from build123d import *

# Parameters (mm, degrees)
CROQUIS1_W              = 138
CROQUIS1_H              = 53
SALIENTE_EXTRUIR1_DEPTH = 5
CROQUIS2_R              = 2.003620998
CROQUIS2_R_2            = 1.5
CROQUIS2_R_3            = 1.25
PRINCIPAL_DEPTH         = 5
CORTAR_EXTRUIR2_DEPTH   = 5
SALIENTE_EXTRUIR2_DEPTH = 5
CORTAR_EXTRUIR3_DEPTH   = 4
CROQUIS6_R              = 4
CORTAR_EXTRUIR4_DEPTH   = 4
SALIENTE_EXTRUIR3_START = 1
CROQUIS8_R              = 1.25
SALIENTE_EXTRUIR3_DEPTH = 1
CROQUIS9_R              = 1
CORTAR_EXTRUIR5_DEPTH   = 10
CROQUIS10_R             = 1
CORTAR_EXTRUIR6_DEPTH   = 10


with BuildPart() as part:
    # Croquis1 → Saliente-Extruir1 (new body)
    with BuildSketch(Plane.XY):
        Rectangle(CROQUIS1_W, CROQUIS1_H)
    extrude(amount=SALIENTE_EXTRUIR1_DEPTH)

    # Croquis2 → Principal (cut)
    with BuildSketch(Plane.XY.offset(5)):
        Polygon((-27.5, -16.5), (-32.5, 10.5), (-27.5, 24.5), (27.5, 24.5), (32.5, 10.5), (27.5, -16.5), align=None)
        with BuildLine():
            Line((-33.613106132, 13.32973033), (-28.909438392, 26.5))
            Line((-28.909438392, 26.5), (-69, 26.5))
            Line((-69, 26.5), (-69, -26.5))
            Line((-69, -26.5), (-29.659776055, -26.5))
            Line((-29.659776055, -26.5), (-46.481481481, 5))
            Line((-46.481481481, 5), (-59.600761168, 5))
            Line((-59.600761168, 5), (-68.394256163, 20.706415948))
            Line((-68.394256163, 20.706415948), (-65.993243243, 22.505064597))
            Line((-65.993243243, 22.505064597), (-57, 10.5))
            Line((-57, 10.5), (-38.5, 10.5))
            ThreePointArc((-38.5, 10.5), (-37, 12), (-35.5, 10.5))
            Line((-35.5, 10.5), (-35.5, 12))
            ThreePointArc((-35.5, 12), (-36.916773994, 15.420394992), (-33.496379002, 14.003620998))
            ThreePointArc((-33.496379002, 14.003620998), (-33.525776447, 13.661658334), (-33.613106132, 13.32973033))
        make_face()
        with BuildLine():
            Line((28.909438392, 26.5), (33.613106132, 13.32973033))
            ThreePointArc((33.613106132, 13.32973033), (35.158037336, 15.977844551), (37.503620998, 14.003620998))
            ThreePointArc((37.503620998, 14.003620998), (36.916773994, 12.586847003), (35.5, 12))
            Line((35.5, 12), (35.5, 10.5))
            ThreePointArc((35.5, 10.5), (37, 12), (38.5, 10.5))
            Line((38.5, 10.5), (57, 10.5))
            Line((57, 10.5), (65.993243243, 22.505064597))
            Line((65.993243243, 22.505064597), (68.394256163, 20.706415948))
            Line((68.394256163, 20.706415948), (59.600761168, 5))
            Line((59.600761168, 5), (46.481481481, 5))
            Line((46.481481481, 5), (29.659776055, -26.5))
            Line((29.659776055, -26.5), (69, -26.5))
            Line((69, -26.5), (69, 26.5))
            Line((69, 26.5), (28.909438392, 26.5))
        make_face()
        with Locations((-35.5, 14.003620998)):
            Circle(CROQUIS2_R)
        with Locations((35.5, 14.003620998)):
            Circle(CROQUIS2_R)
        with Locations((37, 10.5)):
            Circle(CROQUIS2_R_2)
        with Locations((-37, 10.5)):
            Circle(CROQUIS2_R_2)
        with Locations((-6, -21.25)):
            Circle(CROQUIS2_R_3)
        with Locations((6, -21.25)):
            Circle(CROQUIS2_R_3)
    extrude(amount=-PRINCIPAL_DEPTH, mode=Mode.SUBTRACT)

    # Croquis3 → Cortar-Extruir2 (cut)
    with BuildSketch(Plane.XY.offset(5)):
        with BuildLine():
            ThreePointArc((32.325878128, -21.50750886), (28.853998723, -25.156220871), (24, -26.5))
            Line((24, -26.5), (29.659776055, -26.5))
            Line((29.659776055, -26.5), (32.325878128, -21.50750886))
        make_face()
        with BuildLine():
            ThreePointArc((60.578021878, 6.745524755), (59.326103094, 5.468546056), (57.600287393, 5))
            Line((57.600287393, 5), (59.600761168, 5))
            Line((59.600761168, 5), (60.578021878, 6.745524755))
        make_face()
        with BuildLine():
            Line((28.909438392, 26.5), (27.147640402, 26.5))
            ThreePointArc((27.147640402, 26.5), (28.587761459, 26.043538926), (29.501995152, 24.840841072))
            Line((29.501995152, 24.840841072), (28.909438392, 26.5))
        make_face()
    cortar_extruir2 = extrude(amount=-CORTAR_EXTRUIR2_DEPTH, mode=Mode.SUBTRACT)

    # Simetría2: Cortar-Extruir2 across plane
    add(cortar_extruir2.mirror(Plane(origin=(0, 0, 0), x_dir=(0, 0, 1), z_dir=(1, 0, 0))), mode=Mode.SUBTRACT)

    # Croquis4 → Saliente-Extruir2 (add)
    with BuildSketch(Plane.XY.offset(5)):
        with BuildLine():
            ThreePointArc((27.651464932, -15.682089366), (27.30767909, -16.268794305), (26.668182947, -16.5))
            Line((26.668182947, -16.5), (27.5, -16.5))
            Line((27.5, -16.5), (27.651464932, -15.682089366))
        make_face()
        with BuildLine():
            ThreePointArc((26.795280804, 24.5), (27.371329386, 24.317415458), (27.737022835, 23.836336061))
            Line((27.737022835, 23.836336061), (27.5, 24.5))
            Line((27.5, 24.5), (26.795280804, 24.5))
        make_face()
        with BuildLine():
            ThreePointArc((57.299985699, 10.900450382), (56.947113406, 10.605698704), (56.49964811, 10.5))
            Line((56.49964811, 10.5), (57, 10.5))
            Line((57, 10.5), (57.299985699, 10.900450382))
        make_face()
    saliente_extruir2 = extrude(amount=-SALIENTE_EXTRUIR2_DEPTH)

    # Simetría3: Saliente-Extruir2 across plane
    add(saliente_extruir2.mirror(Plane(origin=(0, 0, 0), x_dir=(0, 0, 1), z_dir=(1, 0, 0))))

    # Croquis5 → Cortar-Extruir3 (cut)
    with BuildSketch(Plane.XY.offset(5)):
        with BuildLine():
            Line((32.208888015, 6.182089238), (28.238577223, -15.257589037))
            ThreePointArc((28.238577223, -15.257589037), (29.881835098, -18.638168181), (33.596848928, -18.066080749))
            Line((33.596848928, -18.066080749), (46.000722714, 5.161173227))
            ThreePointArc((46.000722714, 5.161173227), (45.970135784, 6.392832223), (44.898097197, 7))
            Line((44.898097197, 7), (33.192170024, 7))
            ThreePointArc((33.192170024, 7), (32.552673831, 6.768794263), (32.208888015, 6.182089238))
        make_face()
    cortar_extruir3 = extrude(amount=-CORTAR_EXTRUIR3_DEPTH, mode=Mode.SUBTRACT)

    # Simetría4: Cortar-Extruir3 across plane
    add(cortar_extruir3.mirror(Plane(origin=(0, 0, 0), x_dir=(0, 0, 1), z_dir=(1, 0, 0))), mode=Mode.SUBTRACT)

    # Croquis6 → Cortar-Extruir4 (cut)
    with BuildSketch(Plane.XY.offset(5)):
        with Locations((-25, -21.5)):
            Circle(CROQUIS6_R)
        with BuildLine():
            Line((25, -17.5), (-25, -17.5))
            ThreePointArc((-25, -17.5), (-22.171572875, -18.671572875), (-21, -21.5))
            ThreePointArc((-21, -21.5), (-22.171572875, -24.328427125), (-25, -25.5))
            Line((-25, -25.5), (25, -25.5))
            ThreePointArc((25, -25.5), (21, -21.5), (25, -17.5))
        make_face()
        with Locations((25, -21.5)):
            Circle(CROQUIS6_R)
    extrude(amount=-CORTAR_EXTRUIR4_DEPTH, mode=Mode.SUBTRACT)

    # Croquis8 → Saliente-Extruir3 (add)
    # profile 1 of 5: a face of its own
    with BuildSketch(Plane.XY.offset(1).offset(SALIENTE_EXTRUIR3_START)):
        with BuildLine():
            Line((4, -18.5), (4, -17.5))
            Line((4, -17.5), (3, -17.5))
            ThreePointArc((3, -17.5), (3.707106781, -17.792893219), (4, -18.5))
        make_face()
    # profile 2 of 5: a face of its own
    with BuildSketch(Plane.XY.offset(1).offset(SALIENTE_EXTRUIR3_START)):
        Polygon((8, -17.5), (4, -17.5), (4, -18.5), (4, -24.5), (4, -25.5), (8, -25.5), (8, -24.5), (8, -18.5), align=None)
        with Locations((6, -21.25)):
            Circle(CROQUIS8_R, mode=Mode.SUBTRACT)
    # profile 3 of 5: a face of its own
    with BuildSketch(Plane.XY.offset(1).offset(SALIENTE_EXTRUIR3_START)):
        with BuildLine():
            Line((9, -17.5), (8, -17.5))
            Line((8, -17.5), (8, -18.5))
            ThreePointArc((8, -18.5), (8.292893219, -17.792893219), (9, -17.5))
        make_face()
    # profile 4 of 5: a face of its own
    with BuildSketch(Plane.XY.offset(1).offset(SALIENTE_EXTRUIR3_START)):
        with BuildLine():
            ThreePointArc((9, -25.5), (8.292893219, -25.207106781), (8, -24.5))
            Line((8, -24.5), (8, -25.5))
            Line((8, -25.5), (9, -25.5))
        make_face()
    # profile 5 of 5: a face of its own
    with BuildSketch(Plane.XY.offset(1).offset(SALIENTE_EXTRUIR3_START)):
        with BuildLine():
            Line((4, -25.5), (4, -24.5))
            ThreePointArc((4, -24.5), (3.707106781, -25.207106781), (3, -25.5))
            Line((3, -25.5), (4, -25.5))
        make_face()
    saliente_extruir3 = extrude(amount=-SALIENTE_EXTRUIR3_DEPTH)

    # Simetría5: Saliente-Extruir3 across plane
    add(saliente_extruir3.mirror(Plane(origin=(0, 0, 0), x_dir=(0, 0, 1), z_dir=(1, 0, 0))))

    # Croquis9 → Cortar-Extruir5 (cut)
    with BuildSketch(Plane(origin=(31.472457495, -23.576671616, 0), x_dir=(0, 0, 1), z_dir=(-0.8003376397714477, 0.5995495495495503, 0))):
        with Locations(Location((2.5, 54.577869542, 0), (0, 0, 270))):
            Circle(CROQUIS9_R)
        with Locations(Location((2.5, 48.577869542, 0), (0, 0, 270))):
            Circle(CROQUIS9_R)
    cortar_extruir5 = extrude(amount=-CORTAR_EXTRUIR5_DEPTH, mode=Mode.SUBTRACT)

    # Simetría6: Cortar-Extruir5 across plane
    add(cortar_extruir5.mirror(Plane(origin=(0, 0, 0), x_dir=(0, 0, 1), z_dir=(1, 0, 0))), mode=Mode.SUBTRACT)

    # Croquis10 → Cortar-Extruir6 (cut)
    with BuildSketch(Plane(origin=(0, 10.5, 0), x_dir=(1, 0, 0), z_dir=(0, 1, 0))):
        with Locations(Location((52.5, -2.5, 0), (0, 0, 270))):
            Circle(CROQUIS10_R)
        with Locations(Location((41.5, -2.5, 0), (0, 0, 270))):
            Circle(CROQUIS10_R)
    cortar_extruir6 = extrude(amount=-CORTAR_EXTRUIR6_DEPTH, mode=Mode.SUBTRACT)

    # Simetría7: Cortar-Extruir6 across plane
    add(cortar_extruir6.mirror(Plane(origin=(0, 0, 0), x_dir=(0, 0, 1), z_dir=(1, 0, 0))), mode=Mode.SUBTRACT)


solid = part.part
Can you work these out from the model? Positions are in its coordinate system, mm. A direction names the side the tool comes from. Coordinates: 2 decimals unless noted, no trailing zeros. Write each loop counter-clockwise with the first axis right and the second up, starting at its lowest first coordinate (ties: lowest second). Pieces come first, ordered by that corner, then holes. Notation, with made-up numbers: (-28, 34.25) -> (24, 34.25) arc R21 ccw to (24, 54.25) -> close; hole circle Ø11 at (65, 54.25). An arc over 180 degrees is marked (long way). Write item = value, one per line.
(1) Imagine slicing it at B-B (y = -10.5). Please give me the cut outline in (x, z), and give its area (3 significant figures).
Verdict:
outline = (-38.2, 0) -> (-28.61, 0) -> (-28.61, 5) -> (-29.12, 5) -> (-29.12, 1) -> (-37.64, 1) -> (-37.64, 5) -> (-38.2, 5) -> close; (28.61, 0) -> (38.2, 0) -> (38.2, 5) -> (37.64, 5) -> (37.64, 1) -> (29.12, 1) -> (29.12, 5) -> (28.61, 5) -> close
area = 27.8 mm^2
(2) Thinking about a two-plate mould opening in X: for faces 1 (the face through (39.5, -8.07, 2.54)), 2 (the face through (-64.431, 13.628, 3.646)), 3 (the face through (30.085, 17.262, 2.535)), which applies, +X half, -X half, draft (parallel to the pull), parting line (faces both ways), or undercut?
Verdict:
face_1 = +X half
face_2 = -X half
face_3 = undercut
(3) Imagine slicing it at A-A (x = 6). Please give me the cut outline in (y, z), and give its area (3 significant figures).
Verdict:
outline = (-26.5, 0) -> (-22.5, 0) -> (-22.5, 2) -> (-25.5, 2) -> (-25.5, 5) -> (-26.5, 5) -> close; (-20, 0) -> (-16.5, 0) -> (-16.5, 5) -> (-17.5, 5) -> (-17.5, 2) -> (-20, 2) -> close; (24.5, 0) -> (26.5, 0) -> (26.5, 5) -> (24.5, 5) -> close
area = 31.0 mm^2
(4) For pin 1 (2.5 mm diameter, centred on x = -52.5, z = 2.5, fed in from -Y); pin 2 (1.5 mm diameter, centred on x = -6, y = -21.25, fed in from +Z); pin 3 (2.5 mm diameter, centred on x = 21.5, y = -22.5, fed in from +Z); pin 4 (2.5 mm diameter, centred on x = -47.5, z = 3, fed in from +Y), each with a flat end and sliding along its axis, tell me the tip position at first contact or that it passes through.
Verdict:
pin_1 = 5
pin_2 = through
pin_3 = 1
pin_4 = 10.5
(5) On a 3-axis mill with a long thin cutter (end or side, diameter ignored), from which of +Z, -Z, +X, -X, +Y, -Y can I reach the whole of each face in a straight line? I mean faces 4 (the face through (-61.707, 16.784, 2.535)), 5 (the face through (64.54, 13.82, 2.54)), 6 (the face through (0, -25.5, 3)). Say none if no direction works.
Verdict:
face_4 = +Z, -Z, +Y
face_5 = +Z, -Z, +X, -Y
face_6 = +Z
(6) If I drill on probe 1 along Y at (x, z) = (-11, 4); probe 2 along Y at (x, z) = (-6, 1.3); probe 3 along X at (y, z) = (9.5, 0.6), over which ranges is the centre line in solid material (lowest first)?
Verdict:
probe_1 = -26.5 to -25.5, -17.5 to -16.5, 24.5 to 26.5
probe_2 = -26.5 to -22.5, -20 to -16.5, 24.5 to 26.5
probe_3 = -62.12 to -38.12, -35.88 to -32.31, 32.31 to 35.88, 38.12 to 62.12
(7) Imagine slicing it at C-C (x = 37). Please give me the cut outline in (y, z).
Verdict:
outline = (-12.75, 0) -> (9, 0) -> (9, 5) -> (7, 5) -> (7, 1) -> (-11.69, 1) -> (-11.69, 5) -> (-12.75, 5) -> close
